Design review of the part built by this model. Coordinates are the model's own, in mm. Give positions to 0.01 mm unless a question says otherwise; leave off trailing zeros. Write each loop counter-clockwise with the first axis right and the second up, starting at its lowest first coordinate (ties: lowest second). Pieces come first, ordered by that corner, then holes. Notation, with made-up numbers: (-22, 71.25) -> (-12, 71.25) arc R31 ccw to (-12, 102.25) -> close; hole circle Ø11 at (14.25, 85). An arc over 180 degrees is marked (long way). Put each result on its own line as item: value. Start each with the question number.
from build123d import *

# Parameters (mm, degrees)
SKETCH_1_W              = 55
SKETCH_1_H              = 20
EXTRUDE_1_DEPTH         = 18
SKETCH_2_R              = 4
CUT_EXTRUDE_1_DEPTH     = 18
HOLE_WIZARD_6_5_6_5_1_D = 6.5


with BuildPart() as part:
    # Эскиз1 → Бобышка-Вытянуть1 (new body)
    with BuildSketch(Plane.XY):
        Rectangle(SKETCH_1_W, SKETCH_1_H)
    extrude(amount=EXTRUDE_1_DEPTH)

    # Эскиз2 → Вырез-Вытянуть1 (cut)
    with BuildSketch(Plane.XY.offset(18)):
        Circle(SKETCH_2_R)
    extrude(amount=-CUT_EXTRUDE_1_DEPTH, mode=Mode.SUBTRACT)

    # Диаметр отверстия Ø6.5 (6.5)1 (through all)
    with Locations(Plane(origin=(0, 10, 0), x_dir=(1, 0, 0), z_dir=(0, 1, 0))):
        with Locations((19.8, -9), (-19.8, -9)):
            Hole(HOLE_WIZARD_6_5_6_5_1_D / 2)


solid = part.part
Q1. Take a section at A-A on y = 0. Give the boundary of the cut face in (x, z), then the cut area to 3 significant figures.
Q2. Take a section at D-D on z = 12.75. Give the boundary of the cut face in (x, y), then the cut area to 3 significant figures.
Q3. To check wall thickness, follow probe 1 along Y at (x, z) = (0, 10.5); probe 2 along X at (y, z) = (-8, 6.25); probe 3 along X at (y, z) = (0.75, 11.25). State the ranges of each line that lie inside material, in increasing order. Write a range as from..to.
Q4. Take a section at B-B on x = 0. Give the boundary of the cut face in (y, z).
Q5. Mouldability with a two-part tool opening along Z and no side actions: class faces 1 (the face through (0, 5, 0)), 2 (the face through (27.5, 0, 9)), 3 (the face through (23.047, -0.14, 8.857)), 4 (the face through (-16.553, -0.14, 8.857)) as +Z half, -Z half, draft (parallel to the pull), parting line (faces both ways), or undercut.
Q6. Take a section at C-C on z = 9. Give the boundary of the cut face in (x, y).
Result:
1. outline: (-27.5, 0) -> (-4, 0) -> (-4, 18) -> (-27.5, 18) -> close; (4, 0) -> (27.5, 0) -> (27.5, 18) -> (4, 18) -> close; hole circle Ø6.5 at (-19.8, 9); hole circle Ø6.5 at (19.8, 9)
1. area: 780 mm^2
2. outline: (-27.5, -10) -> (27.5, -10) -> (27.5, 10) -> (-27.5, 10) -> close; hole circle Ø8 at (0, 0)
2. area: 1,050 mm^2
3. probe 1: y = -10..-4, 4..10
3. probe 2: x = -27.5..-21.53, -18.07..18.07, 21.53..27.5
3. probe 3: x = -27.5..-22.15, -17.45..-3.93, 3.93..17.45, 22.15..27.5
4. outline: (-10, 0) -> (-4, 0) -> (-4, 18) -> (-10, 18) -> close; (4, 0) -> (10, 0) -> (10, 18) -> (4, 18) -> close
5. face 1: -Z half
5. face 2: draft
5. face 3: undercut
5. face 4: undercut
6. outline: (-27.5, -10) -> (-23.05, -10) -> (-23.05, 10) -> (-27.5, 10) -> close; (-16.55, -10) -> (16.55, -10) -> (16.55, 10) -> (-16.55, 10) -> close; (23.05, -10) -> (27.5, -10) -> (27.5, 10) -> (23.05, 10) -> close; hole circle Ø8 at (0, 0)
